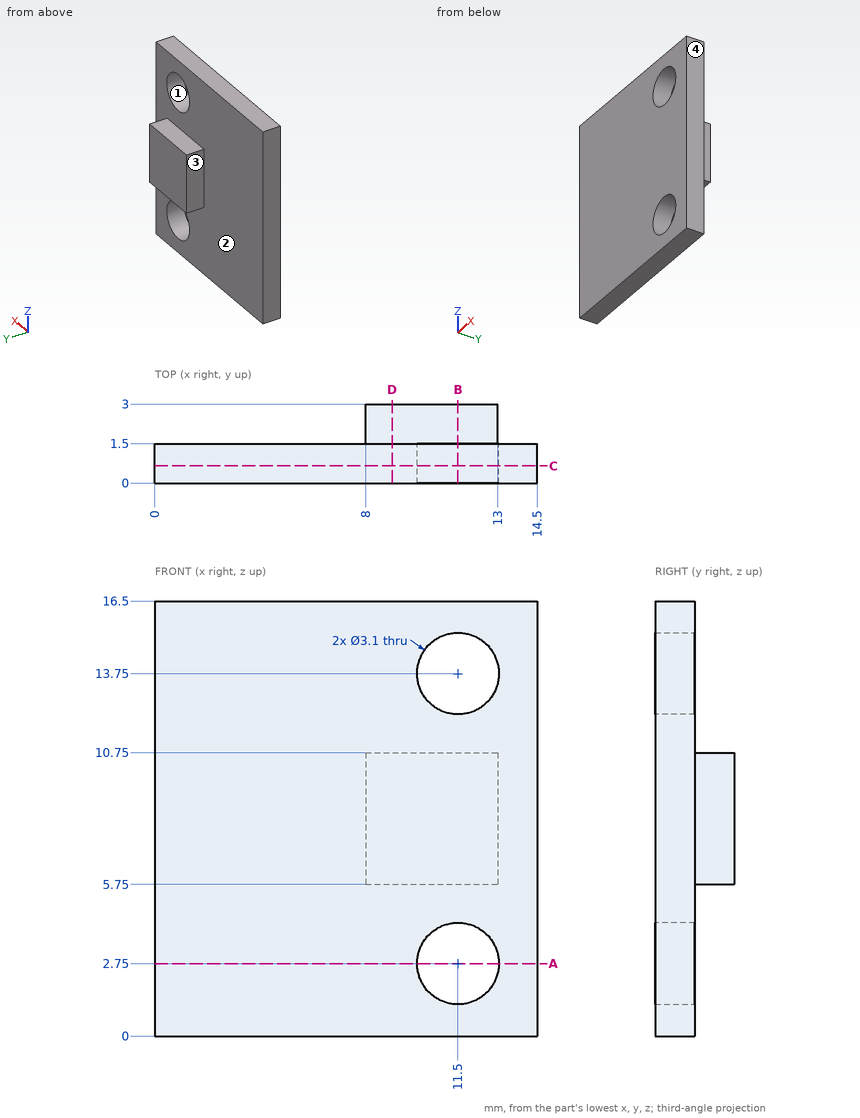
The drawing under review shows one solid part. Ordinate dimensions are in mm from its lowest x, y, z. Coordinates: 2 decimals unless noted, no trailing zeros. Write each loop counter-clockwise with the first axis right and the second up, starting at its lowest first coordinate (ties: lowest second). Pieces come first, ordered by that corner, then holes.
1) Add section C-C (y = 0.65). Write out the cut boundary in (x, z), plus the area to 3 significant figures.
2) To check wall thickness, follow L1, parallel to X at y = 0.7, z = 13.75; L2, parallel to X at y = 2.5, z = 8; L3, parallel to Y at x = 3, z = 4.75. State the ranges of each line that lie inside material, in increasing order.
3) Add section B-B (x = 11.5). Write out the cut boundary in (y, z).
4) Add section A-A (z = 2.75). Write out the cut boundary in (x, y).
5) Insertion check: pin 1 (0.8 mm diameter, centred on y = 2, z = 9, fed in from -X); pin 2 (1.6 mm diameter, centred on y = 2.5, z = 8, fed in from +X). Each pin has a flat end and moves straight along its axis. Give the tip position at first contact, or say it passes through.
6) Add section D-D (x = 9). Write out the cut boundary in (y, z), plus the area to 4 significant figures.
7) Mouldability with a two-part tool opening along X and no side actions: class the marked faces 1, 2, 3 and 4 as +X half, -X half, draft (parallel to the pull), parting line (faces both ways), or undercut.
Check result:
1. outline: (0, 0) - (14.5, 0) - (14.5, 16.5) - (0, 16.5) - close; hole circle Ø3.1 at (11.5, 2.75); hole circle Ø3.1 at (11.5, 13.75)
1. area: 224 mm2
2. L1: x = 0 to 9.95, 13.05 to 14.5
2. L2: x = 8 to 13
2. L3: y = 0 to 1.5
3. outline: (0, 0) - (1.5, 0) - (1.5, 1.2) - (0, 1.2) - close; (0, 4.3) - (1.5, 4.3) - (1.5, 5.75) - (3, 5.75) - (3, 10.75) - (1.5, 10.75) - (1.5, 12.2) - (0, 12.2) - close; (0, 15.3) - (1.5, 15.3) - (1.5, 16.5) - (0, 16.5) - close
4. outline: (0, 0) - (9.95, 0) - (9.95, 1.5) - (0, 1.5) - close; (13.05, 0) - (14.5, 0) - (14.5, 1.5) - (13.05, 1.5) - close
5. pin 1: stops at x = 8
5. pin 2: stops at x = 13
6. outline: (0, 0) - (1.5, 0) - (1.5, 5.75) - (3, 5.75) - (3, 10.75) - (1.5, 10.75) - (1.5, 16.5) - (0, 16.5) - close
6. area: 32.25 mm2
7. face 1: undercut
7. face 2: draft
7. face 3: -X half
7. face 4: +X half
